Study the drawing (mm; zero at the part's minimum x, y, z) and answer. A direction names the side the tool comes from. Give positions to 0.01 mm unless a question says otherwise; leave off trailing zeros. Order: outer loops, then holes, each group sorted by start corner. A loop starts at its lowest first (then second) coordinate and runs counter-clockwise, first axis right, second up. Notation, with made-up numbers: (48.25, 38) - (97.25, 38) arc R10 cw to (97.25, 54) - close; hole circle Ø6 at (18, -27.75). An arc over 180 degrees is marked (long way). Use CSV: the item, a comma, the result in double quotes.
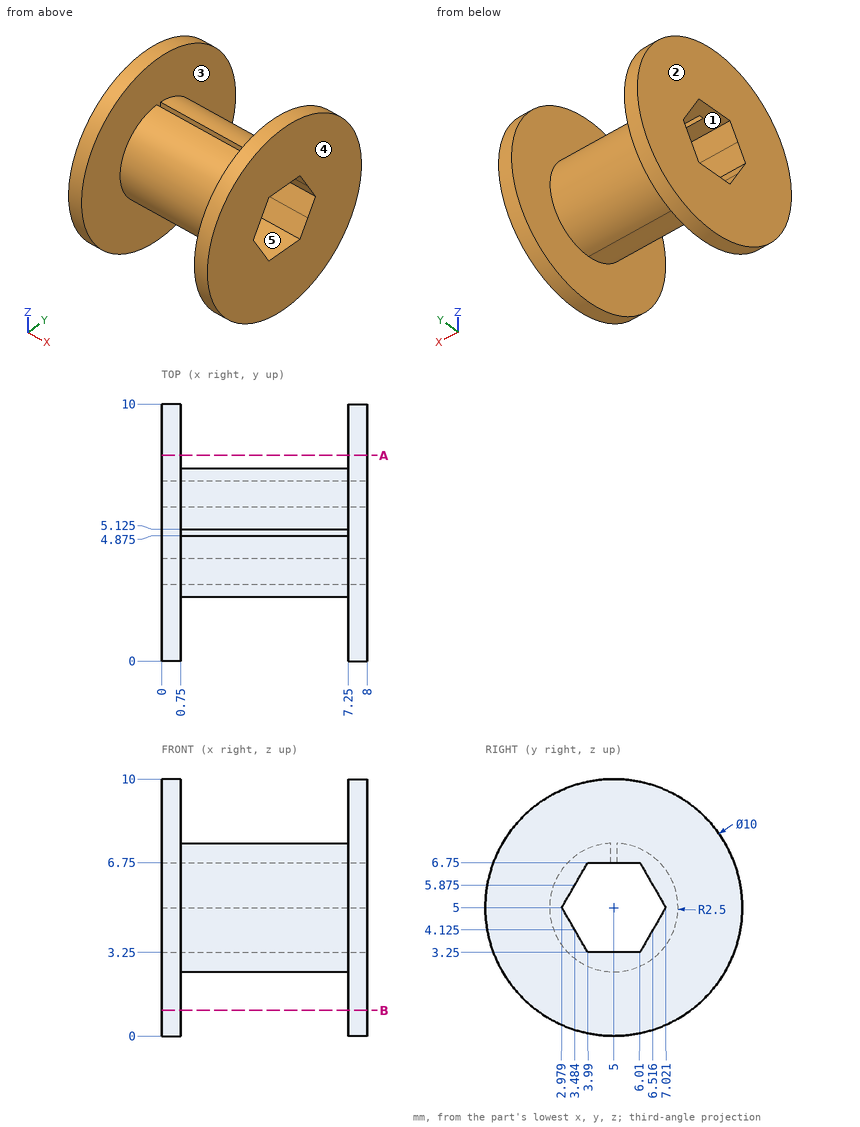
Item 1: The part is cut by section B-B (z = 1). Give the vertices of the cut face in (x, y).
Taken from the geometry:
outline,"(0, 2) - (0.75, 2) - (0.75, 8) - (0, 8) - close; (7.25, 2) - (8, 2) - (8, 8) - (7.25, 8) - close"
Item 2: The part is cut by section A-A (y = 8). Give the vertices of the cut face in (x, z), and give its area (3 significant figures).
Taken from the geometry:
outline,"(0, 1) - (0.75, 1) - (0.75, 9) - (0, 9) - close; (7.25, 1) - (8, 1) - (8, 9) - (7.25, 9) - close"
area,"12.0 mm^2"
Item 3: Find the intervals of material crossed by line 1 along X through (y, z) = (2.5, 5.5); line 2 along Y through (x, z) = (3, 6.5) (1 decimal); line 3 along Y through (x, z) = (3, 6) (1 decimal), in increasing order.
Taken from the geometry:
line 1,"0 to 0.75, 7.25 to 8"
line 2,"3 to 3.8, 6.2 to 7"
line 3,"2.7 to 3.6, 6.4 to 7.3"
Item 4: Which of the six approach directions +Z, -Z, +X, -X, +Y, -Y give full straight-line access (tool end or side, diameter ignored) to the marked faces 1, 2 and 3?
Taken from the geometry:
face 1,"+X, -X"
face 2,"+Z, -Z, -X, +Y, -Y"
face 3,"none"
Item 5: Each of these flat-tipped pins is pushed along its axis until it touches: pin 1 (0.6 mm diameter, centred on x = 4.5, z = 7, fed in from -Y); pin 2 (4 mm diameter, centred on x = 2, y = 8.5, fed in from -Z); pin 3 (1.6 mm diameter, centred on x = 2, y = 5, fed in from +Z). Where does it stop, or does it pass through?
Taken from the geometry:
pin 1,"y = 3.17"
pin 2,"z = 0.39"
pin 3,"z = 7.5"
Item 6: The mould has two halves that part along Y. Classify the marked faces 4 and 5: +Y half, -Y half, draft (parallel to the pull), parting line (faces both ways), or undercut.
Taken from the geometry:
face 4,"draft"
face 5,"undercut"
